Design review of the part built by this model. Coordinates are the model's own, in mm. Round coordinates to 2 decimals unless told otherwise and drop trailing zeros. Order: outer loops, then holes, each group sorted by start corner. A loop starts at its lowest first (then second) coordinate and runs counter-clockwise, first axis right, second up. Notation, with made-up numbers: (-27.75, 82) - (-0.75, 82) arc R18 cw to (-0.75, 108) - close; hole circle Ø5 at (-1, 27). An arc over 180 degrees is marked (long way). Write item = value, one per line.
from build123d import *

# Parameters (mm, degrees)
SKETCH1_W                = 6.5
SKETCH1_H                = 6.5
BOSS_EXTRUDE1_DEPTH      = 18
SKETCH2_W                = 5
SKETCH2_H                = 5
BOSS_EXTRUDE2_DEPTH      = 18.01
BOSS_EXTRUDE2_DEPTH_BACK = 0.01
SWEEP2_PROFILE_R         = 0.35
FILLET2_R                = 0.5


with BuildPart() as part:
    # Sketch1 → Boss-Extrude1 (new body)
    with BuildSketch(Plane(origin=(0, 0, 0), x_dir=(1, 0, 0), z_dir=(0, 1, 0))):
        Rectangle(SKETCH1_W, SKETCH1_H)
    boss_extrude1 = extrude(amount=BOSS_EXTRUDE1_DEPTH)

    # Sketch2 → Boss-Extrude2 (add, two sides)
    with BuildSketch(Plane(origin=(0, 0, 0), x_dir=(1, 0, 0), z_dir=(0, 1, 0))) as boss_extrude2_sk:
        Rectangle(SKETCH2_W, SKETCH2_H)
    extrude(amount=BOSS_EXTRUDE2_DEPTH)
    extrude(boss_extrude2_sk.sketch, amount=-BOSS_EXTRUDE2_DEPTH_BACK)

    # Sweep2: sweep along a path in Sketch4
    with BuildLine(Plane.XY) as sweep2_path:
        Line((3.2, 13), (3.25, 13))
        Line((3.25, 13), (3.75, 13))
        ThreePointArc((3.75, 13), (4.457106781, 12.707106781), (4.75, 12))
        Line((4.75, 12), (4.75, -68.117103267))
    # Sweep2 profile (on start of the path) → Sweep2 (sweep)
    with BuildSketch(Plane(origin=(3.2, 13, 0), x_dir=(0, 0, 1), z_dir=(1, 0, 0))):
        Circle(SWEEP2_PROFILE_R)
    sweep2 = sweep(path=sweep2_path.line)

    # Mirror1: Boss-Extrude1, Sweep2 across plane
    add(boss_extrude1.mirror(Plane(origin=(0, 0, 0), x_dir=(0, 0, 1), z_dir=(1, 0, 0))))
    add(sweep2.mirror(Plane(origin=(0, 0, 0), x_dir=(0, 0, 1), z_dir=(1, 0, 0))))

    # Fillet2
    fillet2_edges = [part.edges().sort_by_distance(p)[0] for p in [
        (3.25, 9, 3.25),
        (-3.25, 9, 3.25),
        (-3.25, 9, -3.25),
        (3.25, 9, -3.25),
    ]]
    fillet(fillet2_edges, radius=FILLET2_R)


solid = part.part
1) To check wall thickness, follow L1, parallel to Y at x = 2.5, z = 0; L2, parallel to Z at x = 4.75, y = -43; L3, parallel to X at y = 5, z = -2.75. State the ranges of each line that lie inside material, in increasing order. Write a range as from..to.
Findings:
L1 = 0..18
L2 = -0.35..0.35
L3 = -3.25..3.25
2) We need section B-B on y = -2. Write out the cut boundary in (x, z), and give its area (3 significant figures).
Findings:
outline = circle Ø0.7 at (-4.75, 0); circle Ø0.7 at (4.75, 0)
area = 0.770 mm^2
3) Clearance check with flat-ended pins moving along their axes: pin 1 Ø1.6 at (y, z) = (10, 1) entering from -X; pin 2 Ø2.5 at (x, z) = (-0.5, 1) entering from -Y. State where each tip first meets the part, or that it passes through.
Findings:
pin_1 = -5.04
pin_2 = -0.01
